Input: part model. Units: mm. Frame: model coordinates. A direction names the side the tool comes from. Give positions to 0.01 mm unless a question says otherwise; leave off trailing zeros. Order: outer loops, then holes, each group sorted by start corner. A loop starts at its lowest first (then second) coordinate and runs counter-clockwise, first axis right, second up. Notation, with made-up numbers: (-24.75, 32.25) - (11.25, 32.25) arc R26 cw to (11.25, 70.25) - close; hole circle Ø6 at (36.5, -9.5). An arc over 180 degrees is marked (long way). Answer in a Markdown table with one row per item. Add a question column.
from build123d import *

# Parameters (mm, degrees)
SKETCH1_R           = 5
BOSS_EXTRUDE1_DEPTH = 10
SKETCH2_W           = 30
SKETCH2_H           = 30
BOSS_EXTRUDE2_DEPTH = 5
BOSS_EXTRUDE3_DEPTH = 5


with BuildPart() as part:
    # Sketch1 → Boss-Extrude1 (new body)
    with BuildSketch(Plane.XY):
        with BuildLine():
            Line((75.304851692, -33.724889915), (25.304851692, -33.724889915))
            Line((25.304851692, -33.724889915), (-6.749247564, -25.10871676))
            ThreePointArc((-6.749247564, -25.10871676), (-25.999433698, 0.171602352), (-6.417227169, 25.195618577))
            Line((-6.417227169, 25.195618577), (25.304851692, 33.275110085))
            Line((25.304851692, 33.275110085), (75.304851692, 33.275110085))
            Line((75.304851692, 33.275110085), (75.304851692, -33.724889915))
        make_face()
        Circle(SKETCH1_R, mode=Mode.SUBTRACT)
    extrude(amount=BOSS_EXTRUDE1_DEPTH)

    # Sketch2 → Boss-Extrude2 (add)
    with BuildSketch(Plane(origin=(75.304851692, 0, 0), x_dir=(0, 0, -1), z_dir=(1, 0, 0))):
        with BuildLine():
            Line((28, 33.275110085), (0, 33.275110085))
            Line((0, 33.275110085), (0, -33.724889915))
            Line((0, -33.724889915), (28, -33.724889915))
            ThreePointArc((28, -33.724889915), (61.5, -0.224889915), (28, 33.275110085))
        make_face()
        with Locations((28, -0.224889915)):
            Rectangle(SKETCH2_W, SKETCH2_H, mode=Mode.SUBTRACT)
    extrude(amount=-BOSS_EXTRUDE2_DEPTH)

    # Sketch3 → Boss-Extrude3 (add)
    with BuildSketch(Plane.XZ.offset(33.724889915)):
        Polygon((70.304851692, -28), (42.304851692, 0), (70.304851692, 0), align=None)
    boss_extrude3 = extrude(amount=-BOSS_EXTRUDE3_DEPTH)

    # Mirror1: Boss-Extrude3 across plane
    add(boss_extrude3.mirror(Plane.ZX.offset(-0.224889915)))


solid = part.part
Q1. Access query for faces 1 (the flat face through (9.502, -29.477, 4.93)), 2 (the flat face through (73, 0, -13)), 3 (the flat face through (60, -28.725, -11)). Directions: +Z, -Z, +X, -X, +Y, -Y. A direction counts if a zero-diameter tool reaches every point of the face in a straight line with its end or side. Return the directions, or none.
Q2. Line query: probe 1 along Y at (x, z) = (67, -10); probe 2 along Z at (x, y) = (64, 24); probe 3 along X at (y, z) = (18, -56). Output: solid intervals per line, ascending.
Q3. Contact query for flat-ended pins moving along their axis: P1, Ø4, axis at y = 23, z = -10.5, coming from the -X side; P2, Ø2.5, axis at x = 73.5, y = -5.5, coming from the -Z side; P3, Ø12, axis at y = -5.5, z = -32, coming from the +X side; P4, Ø1.5, axis at x = 72, z = -35.5, coming from the +Y side. Output: stop coordinate, or through.
Q4. Section B-B, the plane z = -30. Return loops of the section in (x, y).
Q5. Section C-C, the plane y = 0. Return loops of the section in (x, z), then the cut area to 3 significant figures.
Q6. Section A-A, the plane x = -1. Return loops of the section in (y, z), then the cut area to 3 significant figures.
Q7. Section D-D, the plane z = -7.5. Return loops of the section in (x, y).
Q8. Pull-direction query (Y, two-part tool) for faces 4 (the flat face through (56.501, 30.81, -14.196)), 5 (the flat face through (56, -33.725, -5)), 6 (the cylindrical face through (-1.08, -4.88, 4.93)); classes: +Y half, -Y half, draft (parallel to the pull), parting line (faces both ways), or undercut.
Computed:
| question | item | result |
|---|---|---|
| 1 | face 1 | +Z, -Z, -X, -Y |
| 1 | face 2 | +X, -X |
| 1 | face 3 | -Z, -X |
| 2 | probe 1 | y = -33.72 to -28.72, 28.28 to 33.28 |
| 2 | probe 2 | z = 0 to 10 |
| 2 | probe 3 | x = 70.3 to 75.3 |
| 3 | P1 | stops at x = 70.3 |
| 3 | P2 | stops at z = -61.26 |
| 3 | P3 | passes through |
| 3 | P4 | stops at y = 32.59 |
| 4 | outline | (70.3, -33.67) - (75.3, -33.67) - (75.3, -15.22) - (70.3, -15.22) - close; (70.3, 14.78) - (75.3, 14.78) - (75.3, 33.22) - (70.3, 33.22) - close |
| 5 | outline | (-26, 0) - (-5, 0) - (-5, 10) - (-26, 10) - close; (5, 0) - (70.3, 0) - (70.3, -13) - (75.3, -13) - (75.3, 10) - (5, 10) - close; (70.3, -61.5) - (75.3, -61.5) - (75.3, -43) - (70.3, -43) - close |
| 5 | area | 1,070 mm^2 |
| 6 | outline | (-26.65, 0) - (-4.9, 0) - (-4.9, 10) - (-26.65, 10) - close; (4.9, 0) - (26.58, 0) - (26.58, 10) - (4.9, 10) - close |
| 6 | area | 434 mm^2 |
| 7 | outline | (49.8, -33.72) - (75.3, -33.72) - (75.3, 33.28) - (49.8, 33.28) - (49.8, 28.28) - (70.3, 28.28) - (70.3, -28.72) - (49.8, -28.72) - close |
| 8 | face 4 | draft |
| 8 | face 5 | -Y half |
| 8 | face 6 | undercut |
